```python
from build123d import *

# Parameters (mm, degrees)
F0_W     = 10
F0_H     = 10
F1_DEPTH = 5
F2_SIZE2 = 4.99999
F2_SIZE  = 4.99999


# Not quite as in the source:
# - a fillet or chamfer is up to 0.001 mm smaller than in the source, because OpenCascade refuses the exact size
# - a feature names something its author has since deleted; it is built from what else it names


with BuildPart() as f1:
    # F0 (on Front) → F1 (new body, symmetric)
    with BuildSketch(Plane.XZ):
        Rectangle(F0_W, F0_H)
    extrude(amount=F1_DEPTH, both=True)

    # F2 (size 5 and 5 in the source; OpenCascade refuses exactly that, so slightly less here)
    f2_edges = [f1.edges().sort_by_distance(p)[0] for p in [
        (0, -5, 5),
        (-5, -5, 0),
        (0, -5, -5),
        (5, -5, 0),
        (0, 5, 5),
        (-5, 5, 0),
        (0, 5, -5),
        (5, 5, 0),
    ]]
    chamfer(f2_edges, length=F2_SIZE, length2=F2_SIZE2)


solid = f1.part
```
The listing builds one solid part. Answer for the finished solid, in the listing's coordinates (mm). Give positions to 0.01 mm unless a question says otherwise; leave off trailing zeros. Write each loop counter-clockwise with the first axis right and the second up, starting at its lowest first coordinate (ties: lowest second). Pieces come first, ordered by that corner, then holes. Notation, with made-up numbers: (75, 62) -> (107, 62) arc R27 ccw to (107, 101) -> close; hole circle Ø11 at (79.25, 89). An arc over 180 degrees is marked (long way). Write item = value, one per line. Start each with the question number.
1) Determine the mould class of faces 1 (the face through (3, -2, 0)), 2 (the face through (-3, 2, 0)), 3 (the face through (0, -2, 3)) for opening direction X: +X half, -X half, draft (parallel to the pull), parting line (faces both ways), or undercut.
2) Straight lines are drawn through the part: line 1 along Y through (x, z) = (-4, -3); line 2 along X through (y, z) = (-0.5, 4); line 3 along Y through (x, z) = (0.25, 4.5). For each, find the intervals that lie inside material, in ascending order.
3) The part is cut by section D-D, the plane y = 1. Determine the outline of the cut face in (x, z), and give its area (3 significant figures).
4) Each of these flat-tipped pins is pushed along its axis until it touches: pin 1 (4 mm diameter, centred on x = -0.5, y = -3.5, fed in from +Z); pin 2 (4 mm diameter, centred on x = 0, z = -2.5, fed in from -Y); pin 3 (2 mm diameter, centred on y = 3, z = 3.5, fed in from +X); pin 4 (5 mm diameter, centred on x = 2.5, y = -0.5, fed in from +Z). Where does it stop, or does it pass through?
5) The part is cut by section C-C, the plane y = -3.75. Determine the outline of the cut face in (x, z).
Solutions:
q1.face_1 = +X half
q1.face_2 = -X half
q1.face_3 = draft
q2.line_1 = -1 to 1
q2.line_2 = -4.5 to 4.5
q2.line_3 = -0.5 to 0.5
q3.outline = (-4, -4) -> (4, -4) -> (4, 4) -> (-4, 4) -> close
q3.area = 64.0 mm²
q4.pin_1 = 3.5
q4.pin_2 = -4.5
q4.pin_3 = through
q4.pin_4 = 5
q5.outline = (-1.25, -1.25) -> (1.25, -1.25) -> (1.25, 1.25) -> (-1.25, 1.25) -> close
